The figure shows three views and two pictorial views of one solid part (mm, origin at its lowest corner). Answer the questions. A direction names the side the tool comes from. Coordinates: 2 decimals unless noted, no trailing zeros. Order: outer loops, then holes, each group sorted by start corner. A loop starts at its lowest first (then second) coordinate and runs counter-clockwise, first axis right, second up. Notation, with made-up numbers: M -19.5,1.25 L 17.5,1.25 A8 ccw 17.5,15.25 Z; hole C 17,-20.5 d7. An arc over 180 degrees is marked long. Write item = value, one per line. Start each with the question number.
Q1. Straight lines are drawn through the part: line 1 along Y through (x, z) = (0.5, 36); line 2 along Y through (x, z) = (1.75, 56.5) (1 decimal); line 3 along Z through (x, y) = (5.25, 41) (1 decimal). For each, find the intervals that lie inside material, in ascending order.
Q2. Find section C-C on x = 3.5. Give the number of separate pieces and of enclosed holes in the cut face, and give its area (3 significant figures).
Q3. A tool of negligible diameter and unlimited length cuts with its end or side. For the marked faces 4 and 5, from which of +Z, -Z, +X, -X, +Y, -Y can it reach the whole face along a straight path? Write none if from no direction.
Q4. Determine the mould class of the marked faces 1, 2 and 3 for opening direction Z: released by +Z, released by -Z, zero draft, split by the parting line, or undercut.
Q5. Find section A-A on y = 35. Give the vertices of the cut face in (x, z).
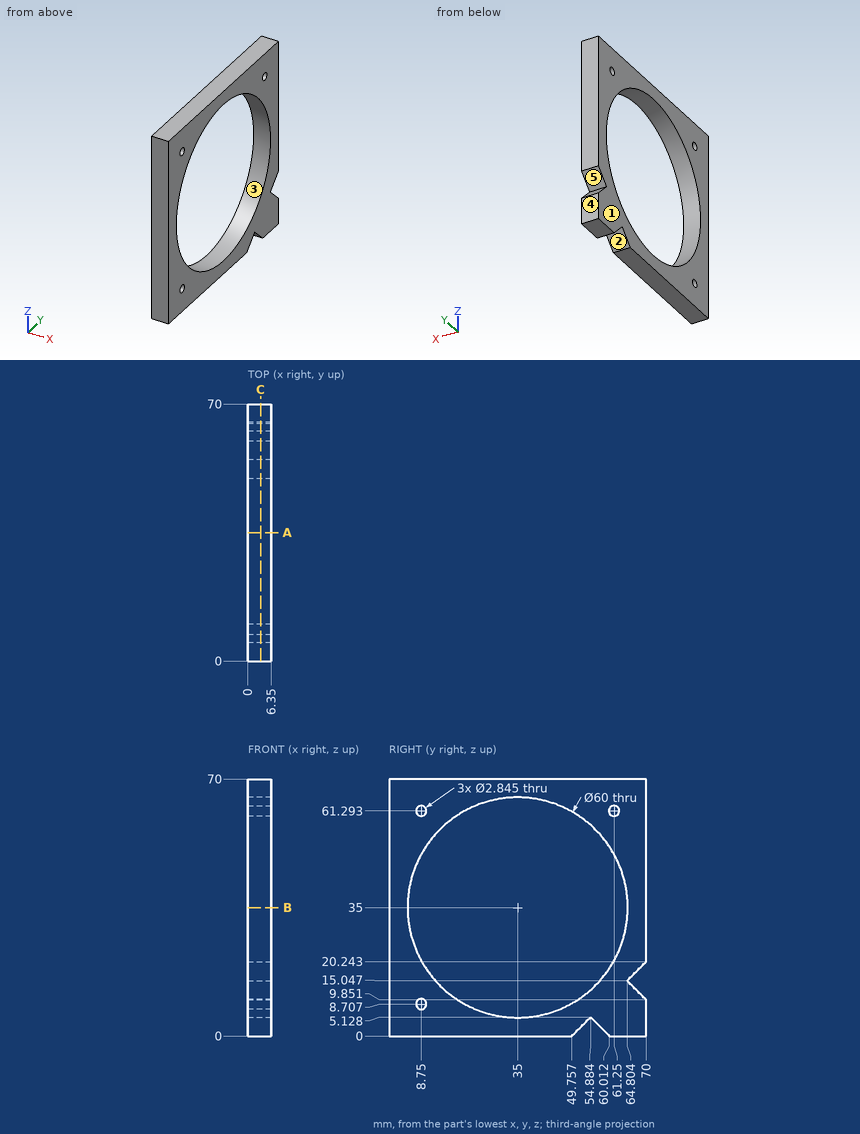
Findings below:
q1.line_1 = 0 to 5.02, 64.98 to 70
q1.line_2 = 0 to 14.1, 55.9 to 70
q1.line_3 = 0 to 5.6, 64.4 to 70
q2.separate_pieces = 1
q2.enclosed_holes = 4
q2.area = 2,000 mm^2
q3.face_4 = +Z, -Z, +X, -X, +Y
q3.face_5 = +X, -X, +Y
q4.face_1 = zero draft
q4.face_2 = released by -Z
q4.face_3 = undercut
q5.outline = M 0,0 L 6.35,0 L 6.35,5 L 0,5 Z; M 0,65 L 6.35,65 L 6.35,70 L 0,70 Z
